from build123d import *

# Parameters (mm, degrees)
F0_R     = 1.4
F1_DEPTH = 20
F2_W     = 21
F2_H     = 10
F2_W_2   = 5
F2_H_2   = 12
F3_DEPTH = 12.5
F4_R     = 1
F5_W     = 5
F5_H     = 12
F6_DEPTH = 25
F7_W     = 5
F7_H     = 12
F8_DEPTH = 25


with BuildPart() as f1:
    # F0 (on Top) → F1 (new body)
    with BuildSketch(Plane.XY):
        with BuildLine():
            ThreePointArc((119.766765, -67.561464), (114.49339, -62.8618), (112.4559, -56.098371))
            Line((112.4559, -56.098371), (112.4552, -42.5148))
            Line((112.4552, -42.5148), (112.4537, -22.9422))
            Line((112.4537, -22.9422), (112.4537, 29.4765))
            Line((112.4537, 29.4765), (113.8864, 47.5783))
            ThreePointArc((113.8864, 47.5783), (114.928823, 50.48122), (117.5795, 52.0584))
            Line((117.5795, 52.0584), (117.197673, 54.021614))
            ThreePointArc((117.197673, 54.021614), (116.964011, 53.943219), (116.719799, 53.909985))
            ThreePointArc((116.719799, 53.909985), (115.899907, 54.156356), (115.407354, 54.85658))
            ThreePointArc((115.407354, 54.85658), (115.379923, 54.971093), (115.362887, 55.087606))
            ThreePointArc((115.362887, 55.087606), (111.760893, 56.708357), (111.084452, 52.816877))
            ThreePointArc((111.084452, 52.816877), (111.1792, 52.726514), (111.270625, 52.632791))
            ThreePointArc((111.270625, 52.632791), (112.084524, 51.250064), (112.222542, 49.651529))
            ThreePointArc((112.222542, 49.651529), (111.978061, 48.670999), (111.886973, 47.664563))
            Line((111.886973, 47.664563), (110.587267, 31.243102))
            Line((110.587267, 31.243102), (110.585941, 31.226352))
            ThreePointArc((110.585941, 31.226352), (110.146932, 30.253847), (109.194256, 29.773325))
            ThreePointArc((109.194256, 29.773325), (109.13192, 29.766581), (109.069367, 29.762284))
            ThreePointArc((109.069367, 29.762284), (106.867452, 27.55672), (108.526545, 24.918472))
            ThreePointArc((108.526545, 24.918472), (108.595788, 24.897473), (108.664459, 24.874672))
            ThreePointArc((108.664459, 24.874672), (109.817927, 24.10839), (110.456089, 22.879396))
            Line((110.456089, 22.879396), (110.456089, 5.614989))
            ThreePointArc((110.456089, 5.614989), (110.460684, 5.47575), (110.456089, 5.336511))
            ThreePointArc((110.456089, 5.336511), (109.982938, 4.13794), (108.901429, 3.43738))
            ThreePointArc((108.901429, 3.43738), (108.8085, 3.414429), (108.714626, 3.395712))
            ThreePointArc((108.714626, 3.395712), (106.8519, 0.977433), (108.716303, -1.439554))
            ThreePointArc((108.716303, -1.439554), (108.804521, -1.457417), (108.891899, -1.479015))
            ThreePointArc((108.891899, -1.479015), (110.005313, -2.215712), (110.456089, -3.47238))
            ThreePointArc((110.456089, -3.47238), (110.456672, -3.522062), (110.456089, -3.571745))
            Line((110.456089, -3.571745), (110.456089, -20.788586))
            ThreePointArc((110.456089, -20.788586), (110.006258, -22.084823), (108.878873, -22.866859))
            ThreePointArc((108.878873, -22.866859), (108.764486, -22.897845), (108.648604, -22.922664))
            ThreePointArc((108.648604, -22.922664), (106.85218, -25.284275), (108.577099, -27.698606))
            ThreePointArc((108.577099, -27.698606), (108.663234, -27.721653), (108.748484, -27.747785))
            ThreePointArc((108.748484, -27.747785), (109.969914, -28.627691), (110.456089, -30.052387))
            ThreePointArc((110.456089, -30.052387), (110.456585, -30.101978), (110.456089, -30.151568))
            Line((110.456089, -30.151568), (110.456089, -47.029801))
            ThreePointArc((110.456089, -47.029801), (109.754616, -48.430568), (108.445892, -49.291647))
            ThreePointArc((108.445892, -49.291647), (106.854026, -51.724792), (108.640977, -54.018487))
            ThreePointArc((108.640977, -54.018487), (109.940136, -54.739828), (110.456206, -56.13332))
            ThreePointArc((110.456206, -56.13332), (111.783653, -62.045742), (115.341962, -66.950565))
            ThreePointArc((115.341962, -66.950565), (115.489565, -67.915475), (115.1972, -68.846797))
            ThreePointArc((115.1972, -68.846797), (115.17136, -68.889542), (115.144539, -68.931677))
            ThreePointArc((115.144539, -68.931677), (116.558423, -72.59606), (119.789896, -70.363493))
            Line((119.789896, -70.363493), (119.946342, -67.869597))
            ThreePointArc((119.946342, -67.869597), (119.903396, -67.688231), (119.766765, -67.561464))
        make_face()
        with Locations((109.3519, -51.6217)):
            Circle(F0_R, mode=Mode.SUBTRACT)
        with Locations((109.3519, -25.3217)):
            Circle(F0_R, mode=Mode.SUBTRACT)
        with Locations((117.2948, -70.206971)):
            Circle(F0_R, mode=Mode.SUBTRACT)
        with Locations((109.3519, 0.9783)):
            Circle(F0_R, mode=Mode.SUBTRACT)
        with Locations((109.3519, 27.2783)):
            Circle(F0_R, mode=Mode.SUBTRACT)
        with Locations((112.9329, 54.5001)):
            Circle(F0_R, mode=Mode.SUBTRACT)
        with BuildLine():
            ThreePointArc((115.1972, -68.846797), (115.170445, -68.888974), (115.144539, -68.931677))
            ThreePointArc((115.144539, -68.931677), (115.17136, -68.889542), (115.1972, -68.846797))
        make_face()
        with BuildLine():
            ThreePointArc((116.719799, 53.909985), (116.964011, 53.943219), (117.197673, 54.021614))
            ThreePointArc((117.197673, 54.021614), (116.957693, 53.970267), (116.719799, 53.909985))
        make_face()
        with BuildLine():
            ThreePointArc((115.362887, 55.087606), (115.379923, 54.971093), (115.407354, 54.85658))
            ThreePointArc((115.407354, 54.85658), (115.38784, 54.972616), (115.362887, 55.087606))
        make_face()
        with BuildLine():
            ThreePointArc((111.270625, 52.632791), (111.1792, 52.726514), (111.084452, 52.816877))
            ThreePointArc((111.084452, 52.816877), (111.175127, 52.722395), (111.270625, 52.632791))
        make_face()
        with BuildLine():
            Line((110.456089, -30.052387), (110.456089, -30.151568))
            ThreePointArc((110.456089, -30.151568), (110.456585, -30.101978), (110.456089, -30.052387))
        make_face()
        with BuildLine():
            ThreePointArc((108.577099, -27.698606), (108.662353, -27.724724), (108.748484, -27.747785))
            ThreePointArc((108.748484, -27.747785), (108.663234, -27.721653), (108.577099, -27.698606))
        make_face()
        with BuildLine():
            ThreePointArc((108.878873, -22.866859), (108.763077, -22.892032), (108.648604, -22.922664))
            ThreePointArc((108.648604, -22.922664), (108.764486, -22.897845), (108.878873, -22.866859))
        make_face()
        with BuildLine():
            ThreePointArc((109.069367, 29.762284), (109.13192, 29.766581), (109.194256, 29.773325))
            ThreePointArc((109.194256, 29.773325), (109.131742, 29.768587), (109.069367, 29.762284))
        make_face()
        with BuildLine():
            Line((110.456089, -3.47238), (110.456089, -3.571745))
            ThreePointArc((110.456089, -3.571745), (110.456672, -3.522062), (110.456089, -3.47238))
        make_face()
        with BuildLine():
            ThreePointArc((108.664459, 24.874672), (108.595788, 24.897473), (108.526545, 24.918472))
            ThreePointArc((108.526545, 24.918472), (108.595185, 24.895574), (108.664459, 24.874672))
        make_face()
        with BuildLine():
            ThreePointArc((108.716303, -1.439554), (108.803746, -1.460865), (108.891899, -1.479015))
            ThreePointArc((108.891899, -1.479015), (108.804521, -1.457417), (108.716303, -1.439554))
        make_face()
        with BuildLine():
            ThreePointArc((110.456089, 5.336511), (110.460684, 5.47575), (110.456089, 5.614989))
            Line((110.456089, 5.614989), (110.456089, 5.336511))
        make_face()
        with BuildLine():
            ThreePointArc((108.901429, 3.43738), (108.807629, 3.418335), (108.714626, 3.395712))
            ThreePointArc((108.714626, 3.395712), (108.8085, 3.414429), (108.901429, 3.43738))
        make_face()
    extrude(amount=F1_DEPTH)

    # F2 (on face) → F3 (cut, symmetric)
    with BuildSketch(Plane(origin=(110.456089, 0, 0), x_dir=(0, -1, 0), z_dir=(-1, 0, 0))):
        with Locations((12.130483, 10)):
            Rectangle(F2_W, F2_H)
        with Locations((-18.493674, 10)):
            Rectangle(F2_W_2, F2_H_2)
        with BuildLine():
            Line((-20.993674, 16), (-15.993674, 16))
            ThreePointArc((-15.993674, 16), (-18.493674, 18.5), (-20.993674, 16))
        make_face()
        with BuildLine():
            ThreePointArc((-20.993674, 4), (-18.493674, 1.5), (-15.993674, 4))
            Line((-15.993674, 4), (-20.993674, 4))
        make_face()
        with Locations((-9.722232, 10)):
            Rectangle(F2_W_2, F2_H_2)
        with BuildLine():
            ThreePointArc((-7.222232, 16), (-9.722232, 18.5), (-12.222232, 16))
            Line((-12.222232, 16), (-7.222232, 16))
        make_face()
        with BuildLine():
            Line((-7.222232, 4), (-12.222232, 4))
            ThreePointArc((-12.222232, 4), (-9.722232, 1.5), (-7.222232, 4))
        make_face()
    extrude(amount=F3_DEPTH, both=True, mode=Mode.SUBTRACT)

    # F4
    f4_edges = [f1.edges().sort_by_distance(p)[0] for p in [
        (110.929494, -22.630483, 5),
        (110.871451, -1.630483, 5),
        (110.871451, -1.630483, 15),
        (110.929494, -22.630483, 15),
    ]]
    fillet(f4_edges, radius=F4_R)

    # F5 (on face) → F6 (cut)
    with BuildSketch(Plane(origin=(107.441437, -8.503649, 0), x_dir=(-0.0789, -0.996883, 0), z_dir=(-0.996883, 0.0789, 0))):
        with Locations((-52.221458, 10)):
            Rectangle(F5_W, F5_H)
        with BuildLine():
            Line((-54.721458, 16), (-49.721458, 16))
            ThreePointArc((-49.721458, 16), (-52.221458, 18.5), (-54.721458, 16))
        make_face()
        with BuildLine():
            ThreePointArc((-54.721458, 4), (-52.221458, 1.5), (-49.721458, 4))
            Line((-49.721458, 4), (-54.721458, 4))
        make_face()
        with BuildLine():
            ThreePointArc((-41.476649, 16), (-43.976649, 18.5), (-46.476649, 16))
            Line((-46.476649, 16), (-41.476649, 16))
        make_face()
        with Locations((-43.976649, 10)):
            Rectangle(F5_W, F5_H)
        with BuildLine():
            Line((-41.476649, 4), (-46.476649, 4))
            ThreePointArc((-46.476649, 4), (-43.976649, 1.5), (-41.476649, 4))
        make_face()
    extrude(amount=-F6_DEPTH, mode=Mode.SUBTRACT)

    # F7 (on face) → F8 (cut)
    with BuildSketch(Plane(origin=(110.456089, 0, 0), x_dir=(0, -1, 0), z_dir=(-1, 0, 0))):
        with Locations((34.29674, 10)):
            Rectangle(F7_W, F7_H)
        with BuildLine():
            Line((31.79674, 16), (36.79674, 16))
            ThreePointArc((36.79674, 16), (34.29674, 18.5), (31.79674, 16))
        make_face()
        with BuildLine():
            ThreePointArc((31.79674, 4), (34.29674, 1.5), (36.79674, 4))
            Line((36.79674, 4), (31.79674, 4))
        make_face()
        with BuildLine():
            ThreePointArc((45.285447, 16), (42.785447, 18.5), (40.285447, 16))
            Line((40.285447, 16), (45.285447, 16))
        make_face()
        with Locations((42.785447, 10)):
            Rectangle(F7_W, F7_H)
        with BuildLine():
            Line((45.285447, 4), (40.285447, 4))
            ThreePointArc((40.285447, 4), (42.785447, 1.5), (45.285447, 4))
        make_face()
    extrude(amount=-F8_DEPTH, mode=Mode.SUBTRACT)


solid = f1.part
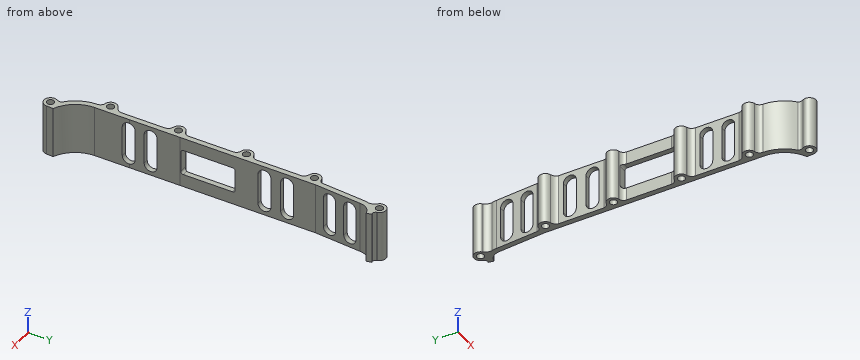
Design review of the part built by this model. Coordinates are the model's own, in mm. Round coordinates to 2 decimals unless told otherwise and drop trailing zeros. Order: outer loops, then holes, each group sorted by start corner. A loop starts at its lowest first (then second) coordinate and runs counter-clockwise, first axis right, second up.
1) Clearance check with flat-ended pins moving along their axes: pin 1 Ø12 at (y, z) = (-38.5, 5) entering from +X; pin 2 Ø3 at (x, z) = (110.5, 18) entering from -Y; pin 3 Ø4 at (y, z) = (-9, 16.5) entering from -X; pin 4 Ø3 at (y, z) = (-6.5, 12) entering from -X. State where each tip first meets the part, or that it passes through.
The answers:
pin 1: stops at x = 112.46
pin 2: stops at y = -62.5
pin 3: stops at x = 110.46
pin 4: passes through
2) Consider section A-A (y = -15.5). State the section outline as (x, z) points, plus the area to 3 significant figures.
The answers:
outline: (110.46, 0) - (112.45, 0) - (112.45, 5) - (110.46, 5) - close; (110.46, 15) - (112.45, 15) - (112.45, 20) - (110.46, 20) - close
area: 20.0 mm2
3) Consider section B-B (z = 8). Count the separate pieces of the cut face and the enclosed holes in it, plus the area to 3 significant figures.
The answers:
separate pieces: 8
enclosed holes: 6
area: 222 mm2
4) For L1, parallel to Y at x = 116.5, z = 14.75; L2, parallel to X at y = -6.5, z = 15.5; L3, parallel to Y at x = 117.75, z = 12.5, list the stretches that pass through material, from the lowest coordinate up.
The answers:
L1: y = -72.58 to -71.36, -69.05 to -65.3, 51.7 to 53.92
L2: x = 110.46 to 112.45
L3: y = -72.67 to -71.53, -68.88 to -66.34
